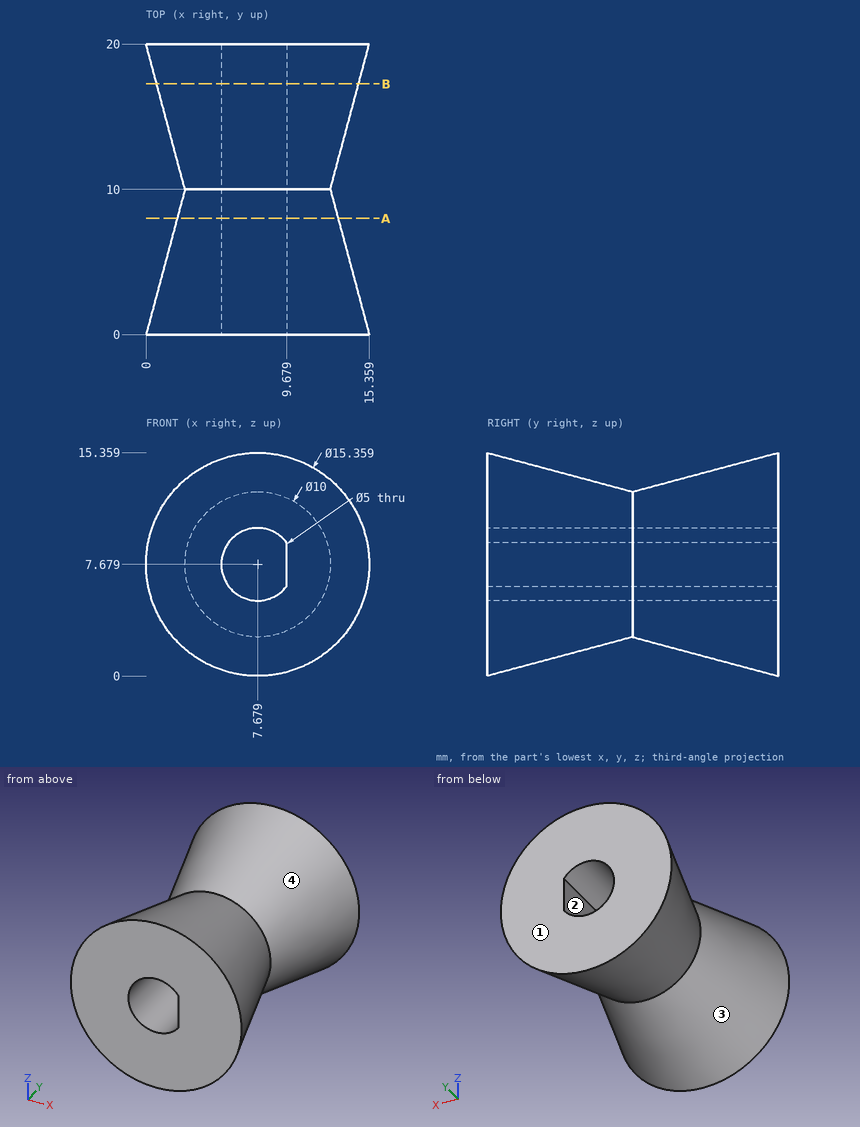
Study the drawing (mm; zero at the part's minimum x, y, z) and answer. Coordinates: 2 decimals unless noted, no trailing zeros. Loops run counter-clockwise (first coordinate to the right, second up) from the corner with the lowest first, then second, coordinate; pieces in that order, holes last. Notation, with made-up numbers: M -38.75,-26 L 14.25,-26 A22 cw 14.25,-1 Z; hole C 44.5,-40 d11. An arc over 180 degrees is marked long. Answer in a Markdown table with one row per item.
1) Find the intervals of material crossed by probe 1 along X at (y, z) = (14.5, 6.5) (1 decimal); probe 2 along Z at (x, y) = (8, 9.5) (1 decimal); probe 3 along Z at (x, y) = (7.5, 8) (1 decimal), in increasing order.
Answers below:
| item | result |
|---|---|
| probe 1 | 1.6 to 5.5, 9.7 to 13.8 |
| probe 2 | 2.6 to 5.2, 10.2 to 12.8 |
| probe 3 | 2.1 to 5.2, 10.2 to 13.2 |
2) Find section B-B (y = 17.25). Determine the outline of the cut face in (x, z) (1 decimal), then the cut area to 3 significant figures.
Answers below:
| item | result |
|---|---|
| outline | C 7.7,7.7 d13.9; hole M 9.7,6.2 L 9.7,9.2 A2.5 ccw long Z |
| area | 133 mm^2 |
3) Find section A-A (y = 8). Determine the outline of the cut face in (x, z) (1 decimal).
Answers below:
| item | result |
|---|---|
| outline | C 7.7,7.7 d11.1; hole M 9.7,6.2 L 9.7,9.2 A2.5 ccw long Z |
4) Given pin 1 (3 mm diameter, centred on x = 6.5, z = 6, fed in from -Y); pin 2 (5 mm diameter, centred on y = 16, z = 4.5, fed in from -X) (1 decimal); pin 3 (8 mm diameter, centred on x = 3.5, y = 5.5, fed in from +Z); pin 4 (1.5 mm diameter, centred on y = 13, z = 8, fed in from -X), each flat-ended and moving along its own axis, determine where each tip first touches the part or whether it passes through.
Answers below:
| item | result |
|---|---|
| pin 1 | y = 0 |
| pin 2 | x = 0.7 |
| pin 3 | z = 14.52 |
| pin 4 | x = 1.68 |
5) Determine the mould class of the marked faces 1, 2, 3 and 4 for opening direction Y: released by +Y, released by -Y, zero draft, split by the parting line, or undercut.
Answers below:
| item | result |
|---|---|
| face 1 | released by +Y |
| face 2 | zero draft |
| face 3 | undercut |
| face 4 | undercut |
